Geometry: final body of the model. Coordinates: model frame, mm. Give positions to 0.01 mm unless a question says otherwise; leave off trailing zeros. Loops run counter-clockwise (first coordinate to the right, second up) from the corner with the lowest first, then second, coordinate; pieces in that order, holes last. Notation, with made-up numbers: (24.5, 29.5) -> (39.5, 29.5) arc R20 cw to (39.5, 37.5) -> close; hole circle Ø6 at (84, 72). An arc over 180 degrees is marked (long way). Answer in a Markdown table with one row per item. Add a question column.
1) Section query B-B (z = 0). Return the cut outline in (x, y).
2) Section query A-A (x = 0). Return the cut outline in (y, z).
3) Line query: line 1 (Z direction, x = 19, y = 0.9); line 2 (X direction, y = 1.3, z = 23). Output: solid intervals per line, ascending. Write a range as from..to.
4) Section query C-C (y = 0.7). Give the number of separate pieces and of enclosed holes in the cut face, plus the area to 3 significant figures.
5) First-contact query: P1, Ø3.5, axis at x = -11, z = 0, coming from the -Y side; P2, Ø1.6, axis at x = -23.5, y = 1, coming from the +Z side; P3, Ø1.5, axis at x = 7, y = 2.5, coming from the +Z side; P4, Ø0.9, axis at x = 20, y = 2, coming from the -Z side. Flat tips, straight axial feed; report the tip coordinate or a pass-through.
6) Section query D-D (z = -17.5). Return the cut outline in (x, y).
```python
from build123d import *

# Parameters (mm, degrees)
SKETCH1_W           = 9
SKETCH1_H           = 9
BOSS_EXTRUDE1_DEPTH = 3
FILLET1_R           = 7
SKETCH2_R           = 6
CUT_EXTRUDE1_DEPTH  = 41.980727178
SKETCH5_R           = 1.4351
CUT_EXTRUDE2_DEPTH  = 41.980727178
CUT_EXTRUDE3_DEPTH  = 41.980727178


with BuildPart() as part:
    # Sketch1 → Boss-Extrude1 (new body)
    with BuildSketch(Plane(origin=(0, 0, 0), x_dir=(1, 0, 0), z_dir=(0, 1, 0))):
        with BuildLine():
            Line((4.5, -24.4), (4.5, -4.5))
            Line((4.5, -4.5), (-4.5, -4.5))
            Line((-4.5, -4.5), (-4.5, -24.4))
            ThreePointArc((-4.5, -24.4), (0, -28.9), (4.5, -24.4))
        make_face()
        Rectangle(SKETCH1_W, SKETCH1_H)
        with BuildLine():
            Line((24.4, 4.5), (4.5, 4.5))
            Line((4.5, 4.5), (4.5, -4.5))
            Line((4.5, -4.5), (24.4, -4.5))
            ThreePointArc((24.4, -4.5), (28.9, 0), (24.4, 4.5))
        make_face()
        with BuildLine():
            Line((4.5, 4.5), (4.5, 24.4))
            ThreePointArc((4.5, 24.4), (0, 28.9), (-4.5, 24.4))
            Line((-4.5, 24.4), (-4.5, 4.5))
            Line((-4.5, 4.5), (4.5, 4.5))
        make_face()
        with BuildLine():
            Line((-4.5, -4.5), (-4.5, 4.5))
            Line((-4.5, 4.5), (-24.4, 4.5))
            ThreePointArc((-24.4, 4.5), (-28.9, 0), (-24.4, -4.5))
            Line((-24.4, -4.5), (-4.5, -4.5))
        make_face()
    extrude(amount=BOSS_EXTRUDE1_DEPTH)

    # Fillet1
    fillet1_edges = [part.edges().sort_by_distance(p)[0] for p in [
        (-4.5, 1.5, 4.5),
        (-4.5, 1.5, -4.5),
        (4.5, 1.5, -4.5),
        (4.5, 1.5, 4.5),
    ]]
    fillet(fillet1_edges, radius=FILLET1_R)

    # Sketch2 → Cut-Extrude1 (cut, through all)
    with BuildSketch(Plane(origin=(0, 3, 0), x_dir=(1, 0, 0), z_dir=(0, 1, 0))):
        with Locations(Location((0, 0, 0), (0, 0, 270))):
            Circle(SKETCH2_R)
    extrude(amount=-CUT_EXTRUDE1_DEPTH, mode=Mode.SUBTRACT)

    # Sketch5 → Cut-Extrude2 (cut, through all)
    with BuildSketch(Plane(origin=(0, 3, 0), x_dir=(1, 0, 0), z_dir=(0, 1, 0))):
        with Locations(Location((-11, 0, 0), (0, 0, 270))):
            Circle(SKETCH5_R)
        with Locations(Location((0, 11, 0), (0, 0, 270))):
            Circle(SKETCH5_R)
        with Locations(Location((11, 0, 0), (0, 0, 270))):
            Circle(SKETCH5_R)
        with Locations(Location((0, -11, 0), (0, 0, 270))):
            Circle(SKETCH5_R)
    extrude(amount=-CUT_EXTRUDE2_DEPTH, mode=Mode.SUBTRACT)

    # Sketch6 → Cut-Extrude3 (cut, through all)
    with BuildSketch(Plane(origin=(0, 3, 0), x_dir=(1, 0, 0), z_dir=(0, 1, 0))):
        with BuildLine():
            Line((-22.4, -2), (-24.4, -2))
            ThreePointArc((-24.4, -2), (-26.4, 0), (-24.4, 2))
            Line((-24.4, 2), (-22.4, 2))
            ThreePointArc((-22.4, 2), (-20.4, 0), (-22.4, -2))
        make_face()
        with BuildLine():
            Line((-2, 22.4), (-2, 24.4))
            ThreePointArc((-2, 24.4), (0, 26.4), (2, 24.4))
            Line((2, 24.4), (2, 22.4))
            ThreePointArc((2, 22.4), (0, 20.4), (-2, 22.4))
        make_face()
        with BuildLine():
            Line((22.4, 2), (24.4, 2))
            ThreePointArc((24.4, 2), (26.4, 0), (24.4, -2))
            Line((24.4, -2), (22.4, -2))
            ThreePointArc((22.4, -2), (20.4, 0), (22.4, 2))
        make_face()
        with BuildLine():
            Line((2, -22.4), (2, -24.4))
            ThreePointArc((2, -24.4), (0, -26.4), (-2, -24.4))
            Line((-2, -24.4), (-2, -22.4))
            ThreePointArc((-2, -22.4), (0, -20.4), (2, -22.4))
        make_face()
    extrude(amount=-CUT_EXTRUDE3_DEPTH, mode=Mode.SUBTRACT)


solid = part.part
```
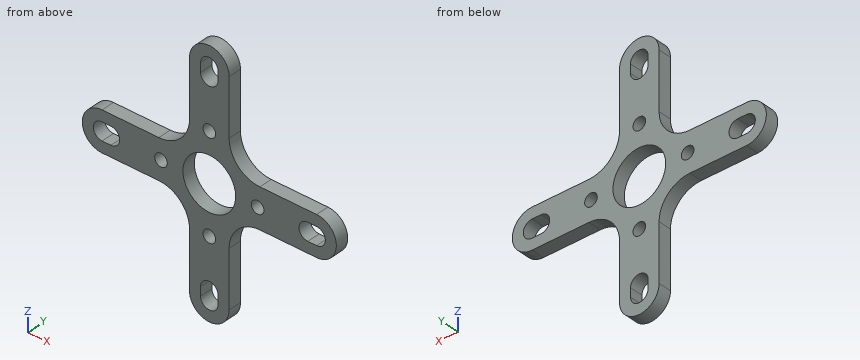
Evaluation:
| question | item | result |
|---|---|---|
| 1 | outline | (-28.9, 0) -> (-26.4, 0) -> (-26.4, 3) -> (-28.9, 3) -> close; (-20.4, 0) -> (-12.44, 0) -> (-12.44, 3) -> (-20.4, 3) -> close; (-9.56, 0) -> (-6, 0) -> (-6, 3) -> (-9.56, 3) -> close; (6, 0) -> (9.56, 0) -> (9.56, 3) -> (6, 3) -> close; (12.44, 0) -> (20.4, 0) -> (20.4, 3) -> (12.44, 3) -> close; (26.4, 0) -> (28.9, 0) -> (28.9, 3) -> (26.4, 3) -> close |
| 2 | outline | (0, -28.9) -> (3, -28.9) -> (3, -26.4) -> (0, -26.4) -> close; (0, -20.4) -> (3, -20.4) -> (3, -12.44) -> (0, -12.44) -> close; (0, -9.56) -> (3, -9.56) -> (3, -6) -> (0, -6) -> close; (0, 6) -> (3, 6) -> (3, 9.56) -> (0, 9.56) -> close; (0, 12.44) -> (3, 12.44) -> (3, 20.4) -> (0, 20.4) -> close; (0, 26.4) -> (3, 26.4) -> (3, 28.9) -> (0, 28.9) -> close |
| 3 | line 1 | -4.5..4.5 |
| 3 | line 2 | -4.5..-2, 2..4.5 |
| 4 | separate pieces | 1 |
| 4 | enclosed holes | 9 |
| 4 | area | 745 mm² |
| 5 | P1 | y = 0 |
| 5 | P2 | z = 4.5 |
| 5 | P3 | z = 6.87 |
| 5 | P4 | z = -4.5 |
| 6 | outline | (-4.5, 0) -> (4.5, 0) -> (4.5, 3) -> (-4.5, 3) -> close |
